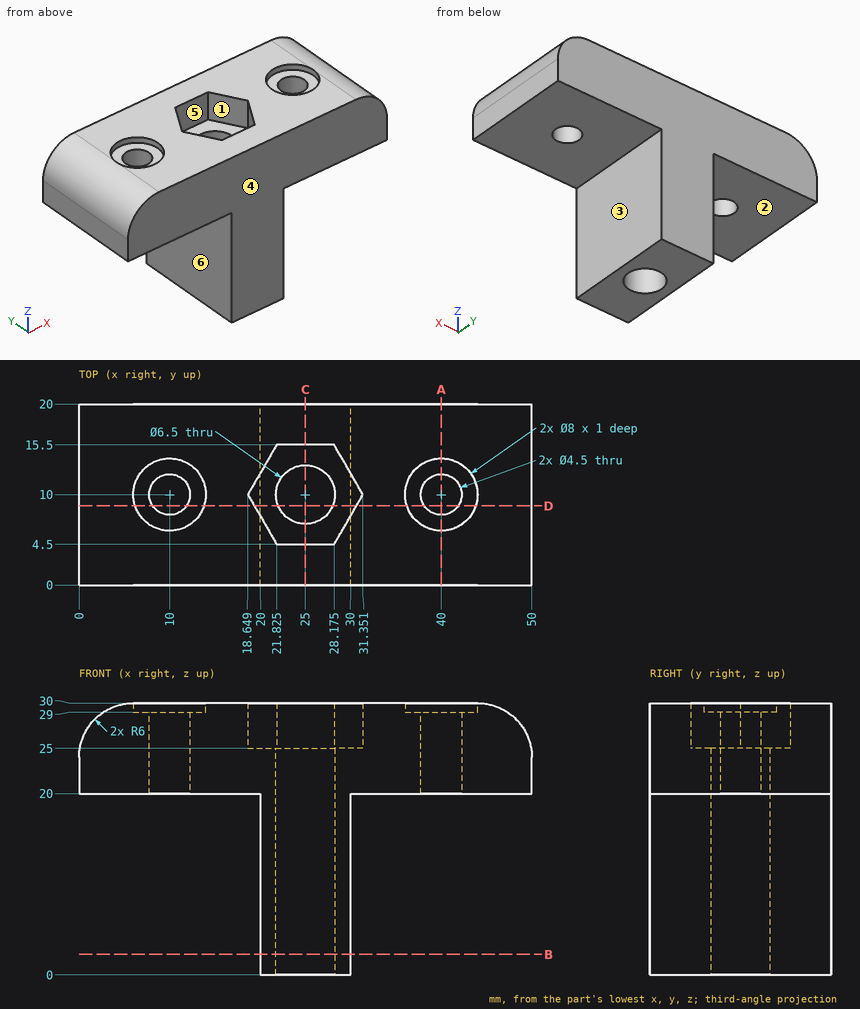
The figure shows three views and two pictorial views of one solid part (mm, origin at its lowest corner). Answer the questions. A direction names the side the tool comes from. Coordinates: 2 decimals unless noted, no trailing zeros. Loops run counter-clockwise (first coordinate to the right, second up) from the corner with the lowest first, then second, coordinate; pieces in that order, holes last. Notation, with made-up numbers: (66, -40) - (77, -40) arc R16 cw to (77, -30) - close; hole circle Ø1 at (-11.75, -24.5). An arc over 180 degrees is marked (long way). Use a Markdown table: item, result. Add a question column.
1) The part is cut by section D-D, the plane y = 8.75. State how many separate pieces and enclosed holes the cut face has, and give its area (3 significant figures).
2) The part is cut by section C-C, the plane x = 25. Give the vertices of the cut face in (y, z).
3) Given pin 1 (10 mm diameter, centred on y = 4, z = 9, fed in from +X); pin 2 (1.5 mm diameter, centred on x = 25.5, z = 27, fed in from -Y); pin 3 (7 mm diameter, centred on x = 40, y = 10, fed in from +Z); pin 4 (6.5 mm diameter, centred on x = 10, y = 10, fed in from -Z), each flat-ended and moving along its own axis, determine where each tip first touches the part or whether it passes through.
4) The mould has two halves that part along Y. Classify the marked faces 4, 5 and 6: released by +Y, released by -Y, zero draft, split by the parting line, or undercut.
5) For the marked faces 1, 2 and 3, determine the directions among +Z, -Z, +X, -X, +Y, -Y from which every point of the face is accessible in a straight line to the end or side of a thin tool.
6) The part is cut by section B-B, the plane z = 2.25. Give the vertices of the cut face in (x, y).
7) Find the intervals of material crossed by line 1 (Y direction, x = 22, z = 28.25); line 2 (Y direction, x = 40, z = 29.3); line 3 (Z direction, x = 27, y = 13.75), in increasing order.
8) The part is cut by section A-A, the plane x = 40. Give the vertices of the cut face in (y, z).
Here are the results:
| question | item | result |
|---|---|---|
| 1 | separate pieces | 4 |
| 1 | enclosed holes | 0 |
| 1 | area | 396 mm^2 |
| 2 | outline | (0, 0) - (6.75, 0) - (6.75, 25) - (4.5, 25) - (4.5, 30) - (0, 30) - close; (13.25, 0) - (20, 0) - (20, 30) - (15.5, 30) - (15.5, 25) - (13.25, 25) - close |
| 3 | pin 1 | stops at x = 30 |
| 3 | pin 2 | stops at y = 0 |
| 3 | pin 3 | stops at z = 29 |
| 3 | pin 4 | stops at z = 20 |
| 4 | face 4 | released by -Y |
| 4 | face 5 | undercut |
| 4 | face 6 | zero draft |
| 5 | face 1 | +Z |
| 5 | face 2 | -Z, -X, +Y, -Y |
| 5 | face 3 | -Z, +X, +Y, -Y |
| 6 | outline | (20, 0) - (30, 0) - (30, 20) - (20, 20) - close; hole circle Ø6.5 at (25, 10) |
| 7 | line 1 | y = 0 to 4.5, 15.5 to 20 |
| 7 | line 2 | y = 0 to 6, 14 to 20 |
| 7 | line 3 | z = 0 to 25 |
| 8 | outline | (0, 20) - (7.75, 20) - (7.75, 29) - (6, 29) - (6, 30) - (0, 30) - close; (12.25, 20) - (20, 20) - (20, 30) - (14, 30) - (14, 29) - (12.25, 29) - close |
